The model under review builds one solid part; all positions refer to its coordinate system, in mm. Coordinates: 2 decimals unless noted, no trailing zeros. Write each loop counter-clockwise with the first axis right and the second up, starting at its lowest first coordinate (ties: lowest second). Pieces come first, ordered by that corner, then holes. Notation, with made-up numbers: (45, 12.25) - (57, 12.25) arc R21 cw to (57, 26.25) - close; hole circle Ø11 at (79, 62.25). An arc over 180 degrees is marked (long way). Put each result on its own line as item: value.
from build123d import *

# Parameters (mm, degrees)
SKETCH1_R      = 65.405
EXTRUDE1_DEPTH = 6.35
SKETCH2_R      = 4.7625
SKETCH2_R_2    = 3.175
EXTRUDE2_DEPTH = 93.714349213


with BuildPart() as part:
    # Sketch1 → Extrude1 (new body)
    with BuildSketch(Plane.XY):
        Circle(SKETCH1_R)
    extrude(amount=EXTRUDE1_DEPTH)

    # Sketch2 → Extrude2 (cut, through all)
    with BuildSketch(Plane.XY.offset(6.35)):
        with Locations((-65.405, 0)):
            Circle(SKETCH2_R)
        with Locations((65.405, 0)):
            Circle(SKETCH2_R)
        with Locations((25.4, 0)):
            Circle(SKETCH2_R_2)
        with Locations((-25.4, 0)):
            Circle(SKETCH2_R_2)
        with BuildLine():
            Line((-25.4, 48.509773864), (-25.4, 60.271502595))
            Line((-25.4, 60.271502595), (-25.4, 90.805))
            Line((-25.4, 90.805), (25.4, 90.805))
            Line((25.4, 90.805), (25.4, 60.271502595))
            Line((25.4, 60.271502595), (25.4, 48.509773864))
            ThreePointArc((25.4, 48.509773864), (0, 23.109773864), (-25.4, 48.509773864))
        make_face()
        with BuildLine():
            Line((20.32, -55.802214755), (20.32, -68.502214755))
            Line((20.32, -68.502214755), (-20.32, -68.502214755))
            Line((-20.32, -68.502214755), (-20.32, -55.802214755))
            ThreePointArc((-20.32, -55.802214755), (0, -35.482214755), (20.32, -55.802214755))
        make_face()
    extrude(amount=-EXTRUDE2_DEPTH, mode=Mode.SUBTRACT)


solid = part.part
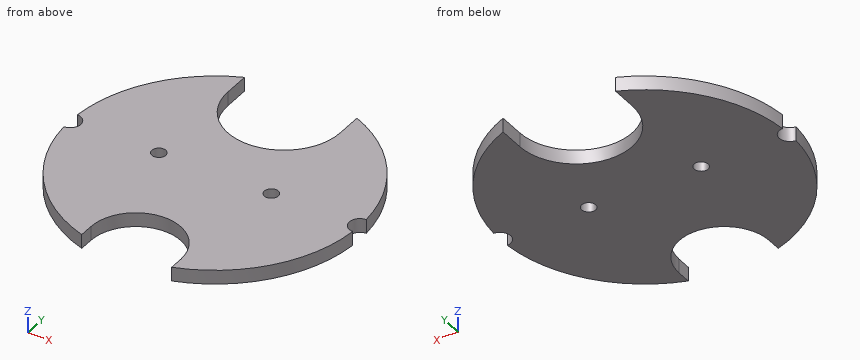
1. For pin 1 Ø3 at (y, z) = (32, 2.5) entering from +X; pin 2 Ø5 at (x, y) = (25.4, 0) entering from -Z; pin 3 Ø2 at (y, z) = (-39.5, 5) entering from +X; pin 4 Ø3 at (x, z) = (-34.5, 5.5) entering from -Y, all flat-tipped, find the tip position at first contact; note any pin that passes through.
Determined:
pin 1: stops at x = 57.86
pin 2: passes through
pin 3: stops at x = 52.87
pin 4: stops at y = -56.47
2. Consider section D-D on x = 0. State the section outline as (y, z) points, plus the area to 3 significant figures.
Determined:
outline: (-35.48, 0) - (23.11, 0) - (23.11, 6.35) - (-35.48, 6.35) - close
area: 372 mm^2
3. Consider section A-A on y = 0. Give the number of separate pieces and of enclosed holes in the cut face, plus the area to 3 significant figures.
Determined:
separate pieces: 3
enclosed holes: 0
area: 690 mm^2
4. Consider section C-C on y = 30.5. State the section outline as (x, z) points.
Determined:
outline: (-57.86, 0) - (-17.91, 0) - (-17.91, 6.35) - (-57.86, 6.35) - close; (17.91, 0) - (57.86, 0) - (57.86, 6.35) - (17.91, 6.35) - close
5. To check wall thickness, follow probe 1 along X at (y, z) = (43, 3.5); probe 2 along X at (y, z) = (-37, 1); probe 3 along X at (y, z) = (5, 4.25). State the ranges of each line that lie inside material, in increasing order.
Determined:
probe 1: x = -49.28 to -24.8, 24.8 to 49.28
probe 2: x = -53.93 to -7.71, 7.71 to 53.93
probe 3: x = -65.21 to 65.21
